Geometry check sheet. Reference: the model listing, model coordinates, mm. A direction names the side the tool comes from. Give positions to 0.01 mm unless a question says otherwise; leave off trailing zeros. Loops run counter-clockwise (first coordinate to the right, second up) from the corner with the lowest first, then second, coordinate; pieces in that order, holes last.
```python
from build123d import *

# Parameters (mm, degrees)
PAD_DEPTH       = 16
SKETCH001_W     = 14.6
SKETCH001_H     = 8.2
POCKET_DEPTH    = 22.001
SKETCH002_W     = 1.6
SKETCH002_H     = 16
POCKET001_DEPTH = 2
CHAMFER_SIZE    = 1.99
POCKET002_DEPTH = 1.601
SKETCH005_R     = 6
SKETCH005_R_2   = 2.8
PAD001_DEPTH    = 3
POCKET003_DEPTH = 7
FILLET_R        = 2
FILLET001_R     = 2
CHAMFER001_SIZE = 1
CHAMFER002_SIZE = 1
SKETCH007_R     = 1.6
POCKET004_DEPTH = 4.5


with BuildPart() as part:
    # Sketch → Pad (new body)
    with BuildSketch(Plane.XY):
        with BuildLine():
            Line((5, 26), (1.6, 26))
            Line((1.6, 26), (1.6, 42))
            Line((1.6, 42), (0, 42))
            Line((0, 42), (0, 0))
            Line((0, 0), (5, 0))
            ThreePointArc((19, 0), (12, 2.206556), (5, 0))
            Line((22, 0), (19, 0))
            Line((22, 26), (22, 0))
            Line((19, 26), (22, 26))
            ThreePointArc((5, 26), (12, 23.793444), (19, 26))
        make_face()
    extrude(amount=PAD_DEPTH)

    # Sketch001 (on Face9 of Pad) → Pocket (cut, through all)
    with BuildSketch(Plane.YZ.offset(22)):
        with Locations((15, 8)):
            Rectangle(SKETCH001_W, SKETCH001_H)
    extrude(amount=-POCKET_DEPTH, mode=Mode.SUBTRACT)

    # Sketch002 (on DatumPlane) → Pocket001 (cut)
    with BuildSketch(Plane.XY.offset(16)):
        with Locations((0.8, 34)):
            Rectangle(SKETCH002_W, SKETCH002_H)
    extrude(amount=-POCKET001_DEPTH, mode=Mode.SUBTRACT)

    # Chamfer
    chamfer_edges = [part.edges().sort_by_distance(p)[0] for p in [
        (0.8, 26, 14),
    ]]
    chamfer(chamfer_edges, length=CHAMFER_SIZE)

    # Sketch003 (on DatumPlane) → Pocket002 (cut, through all)
    with BuildSketch(Plane.YZ.offset(1.6)):
        Polygon((33.7, 14), (35.7, 14), (35.5, 10), (33.9, 10), align=None)
        Polygon((38.7, 14), (39.9, 14), (39.6, 10), (39, 10), align=None)
    extrude(amount=-POCKET002_DEPTH, mode=Mode.SUBTRACT)

    # Sketch005 (on DatumPlane) → Pad001 (join)
    with BuildSketch(Plane.XY.offset(16)):
        with Locations((11, 15)):
            Circle(SKETCH005_R)
        with Locations((11, 15)):
            Circle(SKETCH005_R_2, mode=Mode.SUBTRACT)
    extrude(amount=PAD001_DEPTH)

    # Sketch006 (on DatumPlane) → Pocket003 (cut)
    with BuildSketch(Plane.XY.offset(16)):
        Polygon((15.849742, 15), (13.424871, 19.2), (8.575129, 19.2), (6.150258, 15), (8.575129, 10.8), (13.424871, 10.8), align=None)
    extrude(amount=-POCKET003_DEPTH, mode=Mode.SUBTRACT)

    # Fillet
    fillet_edges = [part.edges().sort_by_distance(p)[0] for p in [
        (5, 15, 16),
    ]]
    fillet(fillet_edges, radius=FILLET_R)

    # Fillet001
    fillet001_edges = [part.edges().sort_by_distance(p)[0] for p in [
        (22, 26, 8),
        (19, 26, 8),
        (5, 26, 8),
        (22, 0, 8),
        (19, 0, 8),
        (5, 0, 8),
    ]]
    fillet(fillet001_edges, radius=FILLET001_R)

    # Chamfer001
    chamfer001_edges = [part.edges().sort_by_distance(p)[0] for p in [
        (0, 15, 12.1),
        (0, 15, 3.9),
        (0, 7.7, 8),
        (0, 22.3, 8),
    ]]
    chamfer(chamfer001_edges, length=CHAMFER001_SIZE)

    # Chamfer002
    chamfer002_edges = [part.edges().sort_by_distance(p)[0] for p in [
        (22, 22.3, 8),
        (22, 15, 12.1),
        (22, 7.7, 8),
        (22, 15, 3.9),
    ]]
    chamfer(chamfer002_edges, length=CHAMFER002_SIZE)

    # Sketch007 (on DatumPlane) → Pocket004 (cut)
    with BuildSketch(Plane.XZ):
        with Locations((1.6, 8)):
            Circle(SKETCH007_R)
    extrude(amount=-POCKET004_DEPTH, mode=Mode.SUBTRACT)


solid = part.part
```
1) Sectioned sample at A-A on y = 25. Enter the section's corners in (x, z).
2) Mould release check, pull along X, two halves, no side actions. Record for faces 1 (the flat face through (3, 26, 8)), 2 (the cylindrical face through (12.097, 2.206, 7.888)), 3 (the flat face through (1.6, 34, 6)): +X half, -X half, draft (parallel to the pull), parting line (faces both ways), or undercut.
3) Sectioned sample at B-B on x = 11. Enter the section's corners in (y, z).
4) Depth check by flat-ended pin: P1, Ø8, axis at y = 15, z = 3.5, coming from the +X side; P2, Ø5, axis at y = 32, z = 5.5, coming from the +X side; P3, Ø0.8, axis at x = 0.5, y = 35, coming from the +Z side; P4, Ø6.5, axis at x = 11.5, z = 9.5, coming from the -Y side. Enter the tip coordinate at first touch or a pass-through.
5) Sectioned sample at D-D on z = 16.5. Enter the section's corners in (x, y).
6) Tool access check on faces 4 (the flat face through (0.811, 38.852, 11.972)), 5 (the flat face through (14.654, 17.071, 14.077)), 6 (the flat face through (11, 7.7, 8)). Record the directions out of +Z, -Z, +X, -X, +Y, -Y that give a thin tool (end or side, any length) a straight path to the whole face; none if there is none.
7) Scan lines: line 1 along Y through (x, z) = (11, 18.35); line 2 along Z through (x, y) = (2.75, 21); line 3 along Z through (x, y) = (11, 9.5). Record each from-to range of solid material in increasing order.
8) Sectioned sample at C-C on y = 13. Count the separate pieces of the cut face and the enclosed holes in it, plus the area to 3 significant figures.
Determined:
1. outline: (0, 0) - (6.71, 0) - (6.71, 16) - (0, 16) - close; (17.29, 0) - (21.73, 0) - (21.73, 16) - (17.29, 16) - close
2. face 1: draft
2. face 2: undercut
2. face 3: +X half
3. outline: (2.17, 0) - (23.83, 0) - (23.83, 16) - (23, 16) arc R2 cw to (21, 18) - (21, 19) - (17.8, 19) - (17.8, 16) - (19.2, 16) - (19.2, 12.1) - (22.3, 12.1) - (22.3, 3.9) - (7.7, 3.9) - (7.7, 12.1) - (10.8, 12.1) - (10.8, 16) - (12.2, 16) - (12.2, 19) - (9, 19) - (9, 18) arc R2 cw to (7, 16) - (2.17, 16) - close
4. P1: stops at x = 22
4. P2: stops at x = 1.6
4. P3: stops at z = 10
4. P4: stops at y = 1.62
5. outline: circle Ø13.35 at (11, 15); hole circle Ø5.6 at (11, 15)
6. face 4: +Z, +X, -X
6. face 5: none
6. face 6: +X, -X
7. line 1: y = 9 to 12.2, 17.8 to 21
7. line 2: z = 0 to 3.9, 12.1 to 16
7. line 3: z = 0 to 3.9, 12.1 to 19
8. separate pieces: 3
8. enclosed holes: 0
8. area: 165 mm2
